Design review of the part shown in the three views and the two pictorial views. Dimensions are in mm from the part's minimum x, y and z. A direction names the side the tool comes from. Coordinates: 2 decimals unless noted, no trailing zeros. Loops run counter-clockwise (first coordinate to the right, second up) from the corner with the lowest first, then second, coordinate; pieces in that order, holes last. Notation, with made-up numbers: (-0.75, 65) - (9.25, 65) arc R27 ccw to (9.25, 90) - close; hole circle Ø3 at (68, 19.25). An arc over 180 degrees is marked (long way). One line per item, written item: value. Start each with the question number.
1. To check wall thickness, follow line 1 (Z direction, x = 155.5, y = 58.5); line 2 (Z direction, x = 87.5, y = 31); line 3 (X direction, y = 35, z = 104.5). State the ranges of each line that lie inside material, in increasing order. Write a range as from..to.
2. Take a section at A-A, the plane y = 57. State the section outline as (x, z) points.
3. Take a section at C-C, the plane z = 117.5. State the section outline as (x, y) points, and give its area (3 significant figures).
4. Take a section at D-D, the plane x = 180. State the section outline as (y, z) points, and give its area (3 significant figures).
5. Take a section at B-B, the plane x = 73.5. State the section outline as (y, z) points, and give its area (3 significant figures).
6. For the marked faces 1 and 2, list the 3-axis set-ups (+Z, -Z, +X, -X, +Y, -Y) from which the entire face can be reached by the end or side of a thin tool; tool diameter is ignored.
7. Insertion check: pin 1 (3 mm diameter, centred on y = 68, z = 110, fed in from -X); pin 2 (6 mm diameter, centred on x = 103, y = 17, fed in from +Z); pin 3 (3 mm diameter, centred on y = 82, z = 96, fed in from +X). Each pin has a flat end and moves straight along its axis. Give the tip position at first contact, or say it passes through.
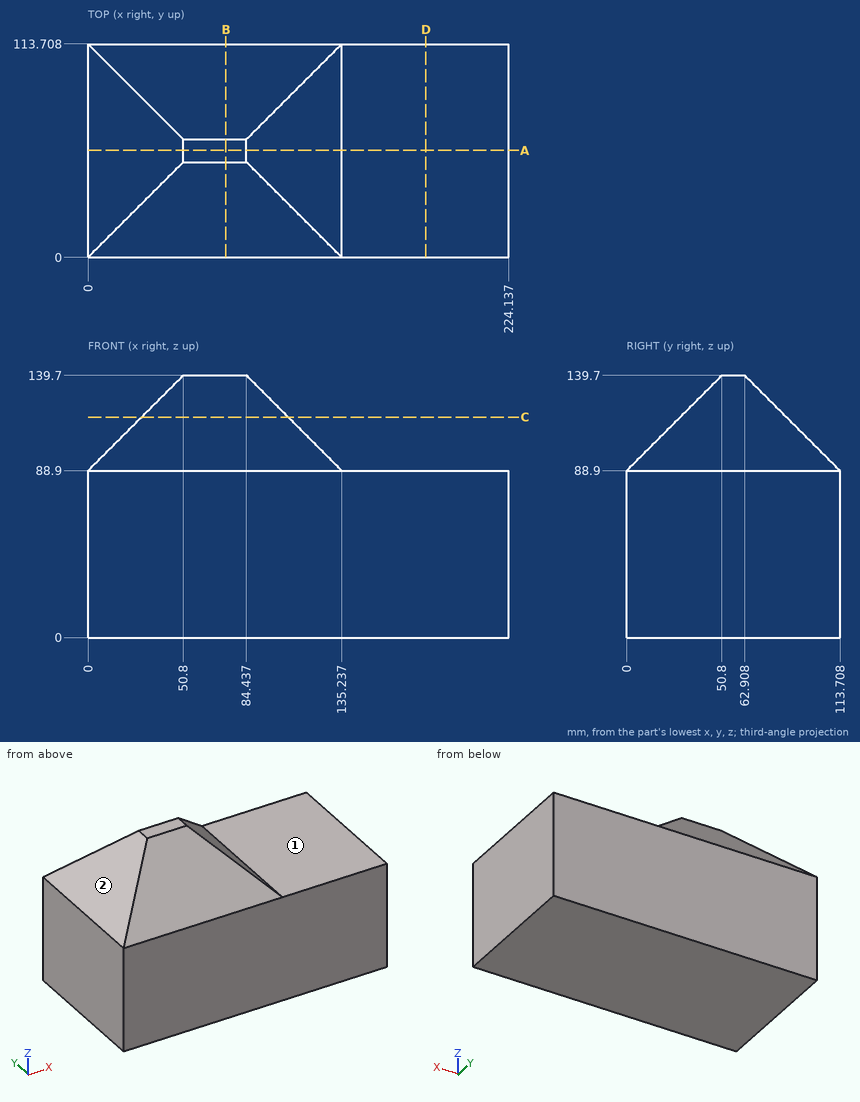
Solutions:
1. line 1: 0..88.9
1. line 2: 0..119.9
1. line 3: 15.6..119.64
2. outline: (0, 0) - (224.14, 0) - (224.14, 88.9) - (135.24, 88.9) - (84.44, 139.7) - (50.8, 139.7) - (0, 88.9) - close
3. outline: (28.6, 28.6) - (106.64, 28.6) - (106.64, 85.11) - (28.6, 85.11) - close
3. area: 4,410 mm2
4. outline: (0, 0) - (113.71, 0) - (113.71, 88.9) - (0, 88.9) - close
4. area: 10,100 mm2
5. outline: (0, 0) - (113.71, 0) - (113.71, 88.9) - (62.91, 139.7) - (50.8, 139.7) - (0, 88.9) - close
5. area: 13,300 mm2
6. face 1: +Z, +X, +Y, -Y
6. face 2: +Z, -X, +Y, -Y
7. pin 1: x = 19.6
7. pin 2: z = 108.9
7. pin 3: x = 129.64
